from build123d import *

# Parameters (mm, degrees)
F0_W           = 5.910679
F0_H           = 19.702202
F1_DEPTH       = 76.2
F3_D           = 6.35
F3_CSINK_D     = 12.7
F3_CSINK_ANGLE = 90
F5_D           = 5
F5_CBORE_D     = 10
F5_CBORE_DEPTH = 1


with BuildPart() as f1:
    # F0 (on Front) → F1 (new body)
    with BuildSketch(Plane.XZ):
        with Locations((85.252292, 27.52936)):
            Rectangle(F0_W, F0_H)
    extrude(amount=F1_DEPTH)

    # F3 (through all)
    with Locations(Plane.XZ.offset(76.2)):
        with Locations((84.467381, 29.080626)):
            CounterSinkHole(F3_D / 2, F3_CSINK_D / 2, counter_sink_angle=F3_CSINK_ANGLE)

    # F5 (through all)
    with Locations(Plane.YZ.offset(88.207632)):
        with Locations((-22.383902, 28.110377)):
            CounterBoreHole(F5_D / 2, F5_CBORE_D / 2, F5_CBORE_DEPTH)


solid = f1.part
Work out the finished part from the listing and answer in its coordinate system (mm). A direction names the side the tool comes from. Give positions to 0.01 mm unless a question says otherwise; leave off trailing zeros. Write each loop counter-clockwise with the first axis right and the second up, starting at its lowest first coordinate (ties: lowest second). Pieces come first, ordered by that corner, then holes. Notation, with made-up numbers: (89, 71) - (145, 71) arc R11 ccw to (145, 77) - close; hole circle Ø6 at (83.25, 46.25). An arc over 180 degrees is marked (long way). One line per item, written item: value. Start each with the question number.
1. For faces 1 (the flat face through (85, 0, 25)), 2 (the cylindrical face through (87.71, -23.47, 23.23)), determine the directions among +Z, -Z, +X, -X, +Y, -Y from which every point of the face is accessible in a straight line to the end or side of a thin tool.
2. For a pull along Z with two mould halves and no side action, classify faces 3 (the cylindrical face through (84.72, -22.34, 25.61)), 4 (the cylindrical face through (87.64, -36, 29.18)), 5 (the flat face through (85, -38, 37.38)), 6 (the flat face through (82.297, -38, 34)) as +Z half, -Z half, draft (parallel to the pull), parting line (faces both ways), or undercut.
3. Find section A-A (y = -34). Write down the section's boundary in (x, z) (3 decimals), then the cut area to 3 significant figures.
4. Consider probe 1 along X at (y, z) = (-35.5, 29.25); probe 2 along Z at (x, y) = (87, -39); probe 3 along Z at (x, y) = (83.9, -18.5). Determine where each line is inside the solid, lowest interval first.
5. Given pin 1 (2 mm diameter, centred on x = 84.5, z = 28, fed in from -Y); pin 2 (1.5 mm diameter, centred on y = -66, z = 28.5, fed in from -X); pin 3 (1.3 mm diameter, centred on y = -22.5, z = 24, fed in from +X), each flat-ended and moving along its own axis, determine where each tip first touches the part or whether it passes through.
Geometry results:
1. face 1: +Z, -Z, +X, -X, +Y
1. face 2: +X
2. face 3: undercut
2. face 4: undercut
2. face 5: +Z half
2. face 6: draft
3. outline: (82.297, 17.678) - (88.208, 17.678) - (88.208, 37.38) - (82.297, 37.38) - (82.297, 31.398) arc R3.175 cw (long way) to (82.297, 26.763) - close
3. area: 88.0 mm2
4. probe 1: 87.64 to 88.21
4. probe 2: 17.68 to 27.17, 31 to 37.38
4. probe 3: 17.68 to 25.96, 32.2 to 37.38
5. pin 1: through
5. pin 2: x = 87.35
5. pin 3: x = 87.21
